Verification items for this drawing (mm, ordinates from the low corner). Coordinates: 2 decimals unless noted, no trailing zeros. Order: outer loops, then holes, each group sorted by start corner. A loop starts at its lowest first (then second) coordinate and runs counter-clockwise, first axis right, second up. Notation, with made-up numbers: M 4,54 L 49,54 A29 ccw 49,77 Z; hole C 61.25,28 d3. An arc over 180 degrees is marked long. Answer as a JSON object with one key per item and string values. Group by question number.
(1) Cross-section at D-D (z = 16). Enter the section's corners in (x, y).
(2) Cross-section at C-C (y = 46.5). Enter the section's corners in (x, z) (1 decimal), plus the area to 3 significant figures.
(3) Gauge pin test, flat ends, axial feed: pin 1 Ø18 at (x, y) = (26.24, 26.24) entering from -Z; pin 2 Ø3 at (y, z) = (14, 7.5) entering from -X; pin 3 Ø5 at (y, z) = (9, 16.5) entering from +X; pin 4 Ø5.5 at (x, y) = (6.24, 26.24) entering from -Z. Record the tip position at first contact, or that the pin passes through.
(4) Material ranges on line 1 (Z direction, x = 24, y = 45); line 2 (X direction, y = 18, z = 4) (1 decimal); line 3 (X direction, y = 19, z = 15.5) (1 decimal), recorded low to high.
(5) Cross-section at A-A (y = 25). Enter the section's corners in (x, z).
(6) Mould release check, pull along Y, two halves, no side actions. Record for the marked faces 1, 2, 3 and 4: released by +Y, released by -Y, zero draft, split by the parting line, or undercut.
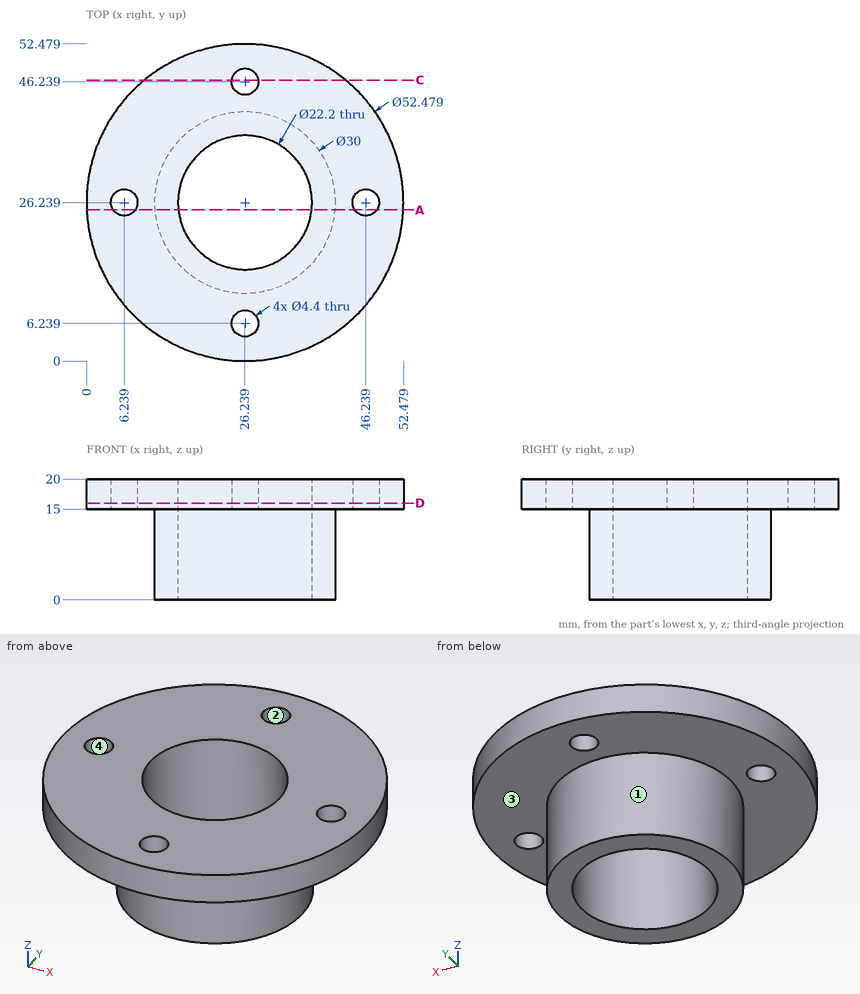
Taken from the geometry:
{
 "1": {"outline": "C 26.24,26.24 d52.48; hole C 6.24,26.24 d4.4; hole C 26.24,26.24 d22.2; hole C 26.24,6.24 d4.4; hole C 26.24,46.24 d4.4; hole C 46.24,26.24 d4.4"},
 "2": {"outline": "M 9.6,15 L 24.1,15 L 24.1,20 L 9.6,20 Z; M 28.4,15 L 42.9,15 L 42.9,20 L 28.4,20 Z", "area": "145 mm²"},
 "3": {"pin 1": "passes through", "pin 2": "stops at x = 15.77", "pin 3": "stops at x = 47.95", "pin 4": "stops at z = 15"},
 "4": {"line 1": "z = 15 to 20", "line 2": "x = 13.7 to 18.8, 33.7 to 38.8", "line 3": "x = 1 to 17.8, 34.7 to 51.5"},
 "5": {"outline": "M 0.03,15 L 4.42,15 L 4.42,20 L 0.03,20 Z; M 8.06,15 L 11.29,15 L 11.29,0 L 15.21,0 L 15.21,20 L 8.06,20 Z; M 37.27,0 L 41.19,0 L 41.19,15 L 44.42,15 L 44.42,20 L 37.27,20 Z; M 48.06,15 L 52.45,15 L 52.45,20 L 48.06,20 Z"},
 "6": {"face 1": "split by the parting line", "face 2": "undercut", "face 3": "zero draft", "face 4": "undercut"}
}
